For this review, use the dimensioned drawing (mm, ordinates from the lowest corner) and the shaded views. A direction names the side the tool comes from. Give positions to 0.01 mm unless a question says otherwise; leave off trailing zeros. Write each loop counter-clockwise with the first axis right and the second up, starting at its lowest first coordinate (ties: lowest second). Pieces come first, ordered by that corner, then holes. Notation, with made-up numbers: M -37,65 L 0,65 A22 ccw 0,89 Z; hole C -12,57.25 d3. An arc over 180 degrees is marked long. One line per item, written item: value. Start each with the question number.
Item 1: To check wall thickness, follow probe 1 along Y at (x, z) = (7.3, 5); probe 2 along Z at (x, y) = (1.5, 8); probe 3 along Z at (x, y) = (7.6, 13.5). State the ranges of each line that lie inside material, in increasing order.
Item 2: Tool access review of the marked faces 1 and 2: name each direction out of +Z, -Z, +X, -X, +Y, -Y from which nothing blocks a thin tool from reaching the whole face with its end or side.
Item 3: Clearance check with flat-ended pins moving along their axes: pin 1 Ø2.5 at (y, z) = (27.5, 5) entering from -X; pin 2 Ø3 at (x, z) = (4, 3.5) entering from +Y. State where each tip first meets the part, or that it passes through.
Item 4: Consider section D-D, the plane x = 5.25. Write out the cut boundary in (y, z).
Item 5: Consider section A-A, the plane z = 5. Write out the cut boundary in (x, y), and give its area (3 significant figures).
Item 6: Consider section C-C, the plane x = 3.25. Write out the cut boundary in (y, z), and give its area (3 significant figures).
Item 7: Consider section B-B, the plane y = 27.5. Write out the cut boundary in (x, z).
Item 8: Mouldability with a two-part tool opening along Z and no side actions: class the marked faces 3, 4, 5 and 6 as released by +Z, released by -Z, zero draft, split by the parting line, or undercut.
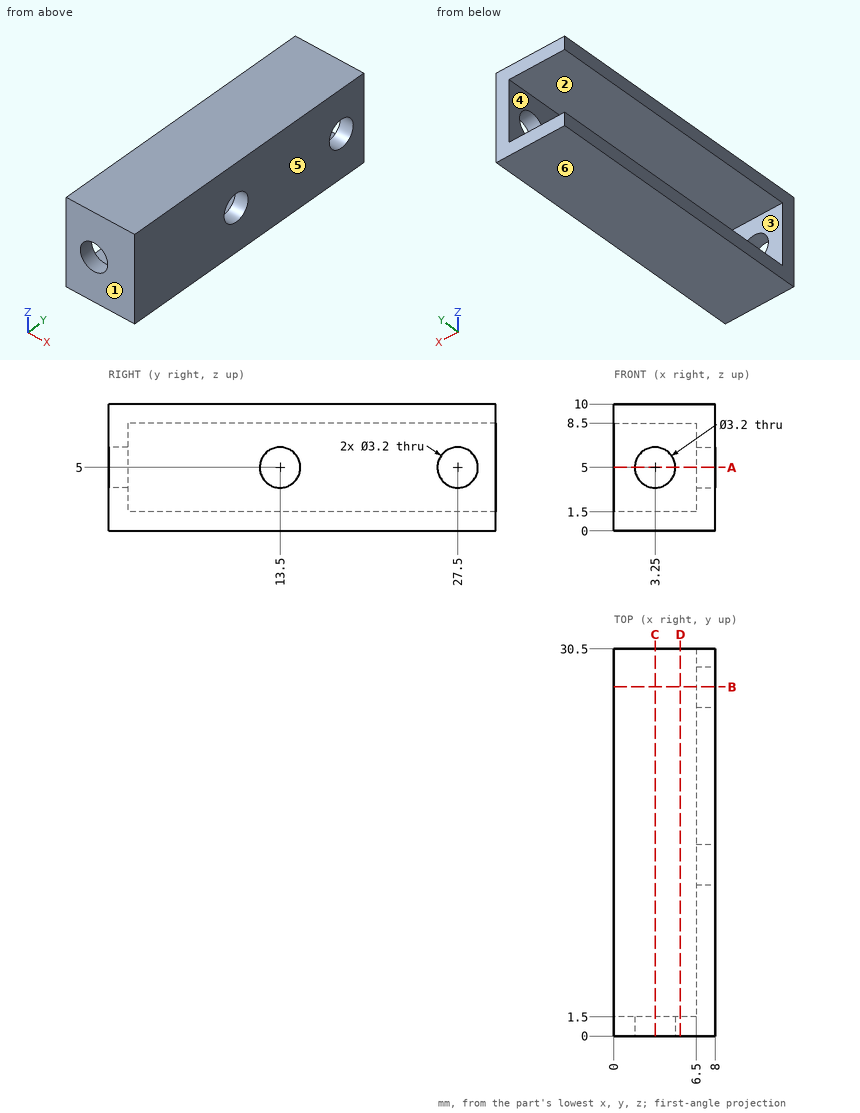
Model answer:
1. probe 1: y = 0 to 11.9, 15.1 to 25.9, 29.1 to 30.5
1. probe 2: z = 0 to 1.5, 8.5 to 10
1. probe 3: z = 0 to 3.4, 6.6 to 10
2. face 1: +Z, -Z, +X, -X, -Y
2. face 2: -X, +Y
3. pin 1: passes through
3. pin 2: stops at y = 1.5
4. outline: M 0,0 L 30.5,0 L 30.5,1.5 L 1.5,1.5 L 1.5,8.5 L 30.5,8.5 L 30.5,10 L 0,10 Z
5. outline: M 0,0 L 1.65,0 L 1.65,1.5 L 0,1.5 Z; M 4.85,0 L 8,0 L 8,11.9 L 6.5,11.9 L 6.5,1.5 L 4.85,1.5 Z; M 6.5,15.1 L 8,15.1 L 8,25.9 L 6.5,25.9 Z; M 6.5,29.1 L 8,29.1 L 8,30.5 L 6.5,30.5 Z
5. area: 41.1 mm2
6. outline: M 0,0 L 30.5,0 L 30.5,1.5 L 1.5,1.5 L 1.5,3.4 L 0,3.4 Z; M 0,6.6 L 1.5,6.6 L 1.5,8.5 L 30.5,8.5 L 30.5,10 L 0,10 Z
6. area: 97.2 mm2
7. outline: M 0,0 L 8,0 L 8,3.4 L 6.5,3.4 L 6.5,1.5 L 0,1.5 Z; M 0,8.5 L 6.5,8.5 L 6.5,6.6 L 8,6.6 L 8,10 L 0,10 Z
8. face 3: undercut
8. face 4: undercut
8. face 5: zero draft
8. face 6: released by -Z
